Geometry check sheet. Reference: drawing and pictorial views, mm from the part's lowest x, y, z. A direction names the side the tool comes from. Round coordinates to 2 decimals unless told otherwise and drop trailing zeros. Order: outer loops, then holes, each group sorted by start corner. A loop starts at its lowest first (then second) coordinate and runs counter-clockwise, first axis right, second up.
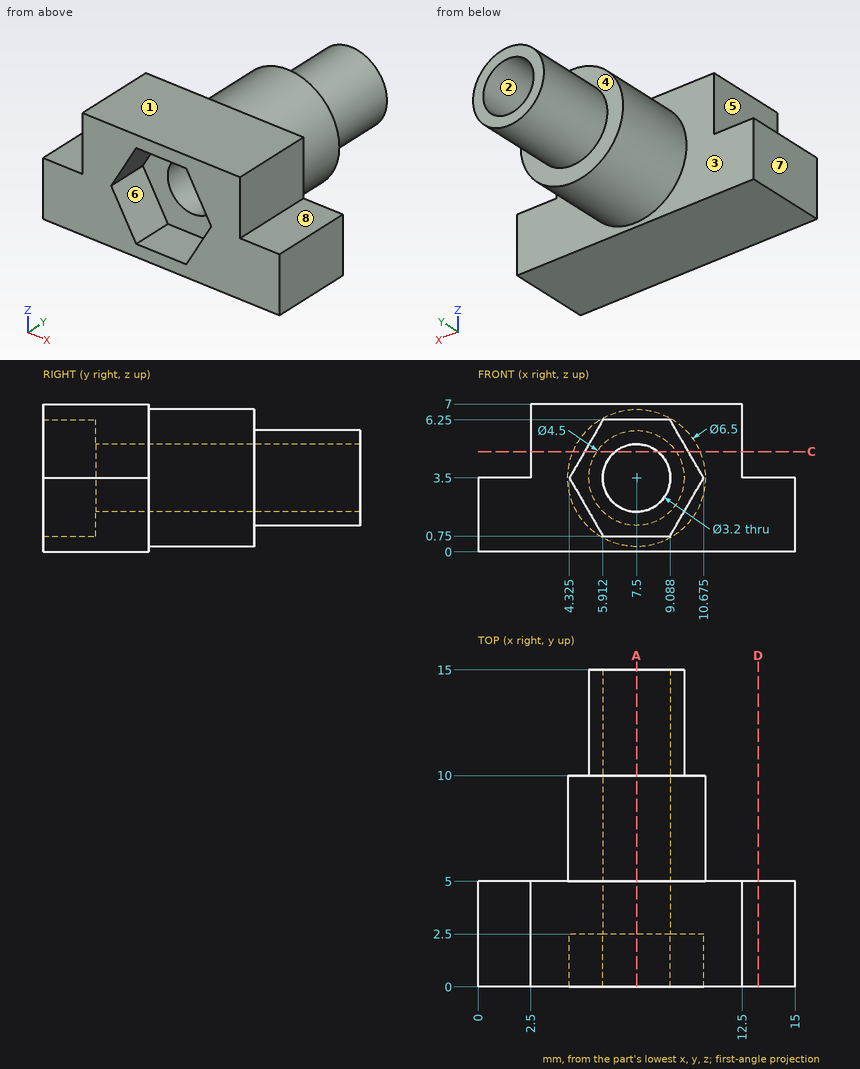
1) Tool access check on the marked faces 4, 5, 6, 7 and 8. Record the directions out of +Z, -Z, +X, -X, +Y, -Y that give a thin tool (end or side, any length) a straight path to the whole face; none if there is none.
2) Go/stop test with flat-tipped pins: pin 1 Ø5 at (x, y) = (6.5, 10.5) entering from -Z; pin 2 Ø4 at (x, y) = (2.5, 10) entering from +Z; pin 3 Ø1.8 at (y, z) = (1.5, 5.5) entering from +X; pin 4 Ø1 at (x, z) = (8, 4) entering from +Y. Record where each tip stops, or that it passes through.
3) Sectioned sample at A-A on x = 7.5. Record the cut outline in (y, z).
4) Sectioned sample at C-C on z = 4.75. Record the cut outline in (x, y).
5) Scan lines: probe 1 along X at (y, z) = (11, 3.5); probe 2 along Z at (x, y) = (6, 1.75); probe 3 along Z at (x, y) = (7.5, 8.25). Record each from-to range of solid material in increasing order.
6) Draft check along Z on the marked faces 1, 2 and 3. Enter one of: released by +Z, released by -Z, zero draft, split by the parting line, or undercut.
7) Sectioned sample at D-D on x = 13.25. Record the cut outline in (y, z), then the cut area to 3 significant figures.
Returned:
1. face 4: +Y
1. face 5: +Z, -X, +Y, -Y
1. face 6: -Y
1. face 7: +Z, -Z, -X, +Y, -Y
1. face 8: +Z, +X, +Y, -Y
2. pin 1: stops at z = 0.25
2. pin 2: stops at z = 4.75
2. pin 3: stops at x = 12.5
2. pin 4: passes through
3. outline: (0, 0) - (5, 0) - (5, 0.25) - (10, 0.25) - (10, 1.25) - (15, 1.25) - (15, 1.9) - (2.5, 1.9) - (2.5, 0.75) - (0, 0.75) - close; (0, 6.25) - (2.5, 6.25) - (2.5, 5.1) - (15, 5.1) - (15, 5.75) - (10, 5.75) - (10, 6.75) - (5, 6.75) - (5, 7) - (0, 7) - close
4. outline: (2.5, 0) - (5.05, 0) - (5.05, 2.5) - (6.5, 2.5) - (6.5, 15) - (5.63, 15) - (5.63, 10) - (4.5, 10) - (4.5, 5) - (2.5, 5) - close; (8.5, 2.5) - (9.95, 2.5) - (9.95, 0) - (12.5, 0) - (12.5, 5) - (10.5, 5) - (10.5, 10) - (9.37, 10) - (9.37, 15) - (8.5, 15) - close
5. probe 1: x = 5.25 to 5.9, 9.1 to 9.75
5. probe 2: z = 0 to 0.75, 6.25 to 7
5. probe 3: z = 0.25 to 1.9, 5.1 to 6.75
6. face 1: released by +Z
6. face 2: undercut
6. face 3: zero draft
7. outline: (0, 0) - (5, 0) - (5, 3.5) - (0, 3.5) - close
7. area: 17.5 mm2
